Autodesk Inventor part; units mm, degrees
ref_plane "YZ Plane" through (0, 0, 0) normal (1, 0, 0) x (0, 1, 0)
ref_plane "XZ Plane" through (0, 0, 0) normal (0, 1, 0) x (-1, 0, 0)
ref_plane "XY Plane" through (0, 0, 0) normal (0, 0, 1) x (1, 0, 0)
sketch "草图1" plane through (0, 0, 0) normal (1, 0, 0) x (0, 1, 0)
  circle A0 centre (0, 0) radius 15 construction
  line L0 (0, 0) -> (0, -15) construction
  circle A1 centre (0, 0) radius 10
  circle A2 centre (0, -15) radius 2.1
  circle A3 centre (12.9904, -7.5) radius 2.1
  circle A4 centre (12.9904, 7.5) radius 2.1
  circle A5 centre (0, 15) radius 2.1
  circle A6 centre (-12.9904, 7.5) radius 2.1
  circle A7 centre (-12.9904, -7.5) radius 2.1
  circle A8 centre (0, 0) radius 20
  dimension "d0" = 30
  dimension "d1" = 20
  dimension "d2" = 4.2
  dimension "d5" = 360
  dimension "d7" = 40
extrude "拉伸1" add sketch "草图1" along normal blind 6
sketch "草图2" plane through (6, 0, 0) normal (1, 0, 0) x (0, 0, -1)
  circle A0 centre (0, 0) radius 4
  circle A1 centre (0, 0) radius 20
  circle A2 centre (15, 0) radius 2.1
  circle A3 centre (15, 0) radius 3.5
  circle A4 centre (7.5, 12.9904) radius 3.5
  circle A5 centre (-7.5, 12.9904) radius 3.5
  circle A6 centre (-15, 0) radius 3.5
  circle A7 centre (-7.5, -12.9904) radius 3.5
  circle A8 centre (7.5, -12.9904) radius 3.5
  dimension "d10" = 8
  dimension "d11" = 7
  dimension "d14" = 360
extrude "拉伸2" add sketch "草图2" along normal blind 5 contours A1
sketch "草图3" plane through (11, 0, 0) normal (1, 0, 0) x (0, 0, -1)
  circle A0 centre (0, 0) radius 4
  circle A1 centre (0, 0) radius 9
  dimension "d18" = 18
extrude "拉伸3" add sketch "草图3" along normal blind 10
chamfer "倒角1" distance 2 angle 45 1 edges at (11, 0, 9)
chamfer "倒角2" distance 1 angle 45 1 edges at (11, 0, 20)
properties part number "链轮摇臂座"
Geometry: final body of the model. Coordinates: model frame, mm. A direction names the side the tool comes from. Round coordinates to 2 decimals unless told otherwise and drop trailing zeros. Write each loop counter-clockwise with the first axis right and the second up, starting at its lowest first coordinate (ties: lowest second). Pieces come first, ordered by that corner, then holes. Notation, with made-up numbers: M -39.5,-17 L -34.5,-17 A30 cw -34.5,20 Z; hole C 80,1.5 d10. An arc over 180 degrees is marked long. Write item = value, one per line.
Item 1: Pull-direction query (Z, two-part tool) for faces 1 (the face through (11, -8, -8)), 2 (the face through (8.46, -1.05, -18.34)); classes: pulls with the +Z half, pulls with the -Z half, needs draft (parallel to the pull), parting line crosses it, or undercut.
Findings:
face_1 = needs draft
face_2 = undercut
Item 2: Access query for faces 3 (the face through (2.958, -0.273, 12.918)), 4 (the face through (8.46, 15.12, -4.72)), 5 (the face through (2.96, -2.17, 9.76)). Directions: +Z, -Z, +X, -X, +Y, -Y. A direction counts if a zero-diameter tool reaches every point of the face in a straight line with its end or side. Return the directions, or none.
Findings:
face_3 = +X, -X
face_4 = +X
face_5 = -X
Item 3: Section query A-A on z = 0. Return loops of the section in (x, y).
Findings:
outline = M 0,-20 L 10,-20 L 11,-19 L 11,-11 L 13,-9 L 21,-9 L 21,-4 L 6,-4 L 6,-10 L 0,-10 Z; M 0,10 L 6,10 L 6,4 L 21,4 L 21,9 L 13,9 L 11,11 L 11,19 L 10,20 L 0,20 Z
Item 4: Section query D-D on x = 12.5. Return loops of the section in (y, z).
Findings:
outline = C 0,0 d19; hole C 0,0 d8
Item 5: Pin query (flat end, axial travel): P1, Ø18, axis at y = 0, z = 0, coming from the -X side; P2, Ø7.5, axis at y = -0.5, z = 14, coming from the +X side; P3, Ø2.5, axis at y = -12.99, z = 7.5, coming from the +X side; P4, Ø1.5, axis at x = 11.5, z = 13, coming from the +Y side. Return the tip coordinate at first contact, or that it passes through.
Findings:
P1 = 6
P2 = 11.74
P3 = through
P4 = 14.4
Item 6: Material intervals for line 1 along Z through (x, y) = (4.75, 0); line 2 along Y through (x, z) = (9.8, 7.5); line 3 along Z through (x, y) = (8.25, 13), sorted ascending. Write a range as [from, to].
Findings:
line_1 = [-20, -17.1], [-12.9, -10], [10, 12.9], [17.1, 20]
line_2 = [-18.54, -16.49], [-9.49, 9.49], [16.49, 18.54]
line_3 = [-15.2, -11], [-4, 4], [11, 15.2]
Item 7: Section query B-B on y = 0. State how many separate pieces and enclosed holes the cut face has, then the cut area to 3 significant figures.
Findings:
separate_pieces = 4
enclosed_holes = 0
area = 263 mm^2
Item 8: Section query C-C on x = 8.75. Return loops of the section in (y, z).
Findings:
outline = C 0,0 d40; hole C -12.99,-7.5 d7; hole C -12.99,7.5 d7; hole C 0,0 d8; hole C 0,-15 d7; hole C 0,15 d7; hole C 12.99,-7.5 d7; hole C 12.99,7.5 d7
